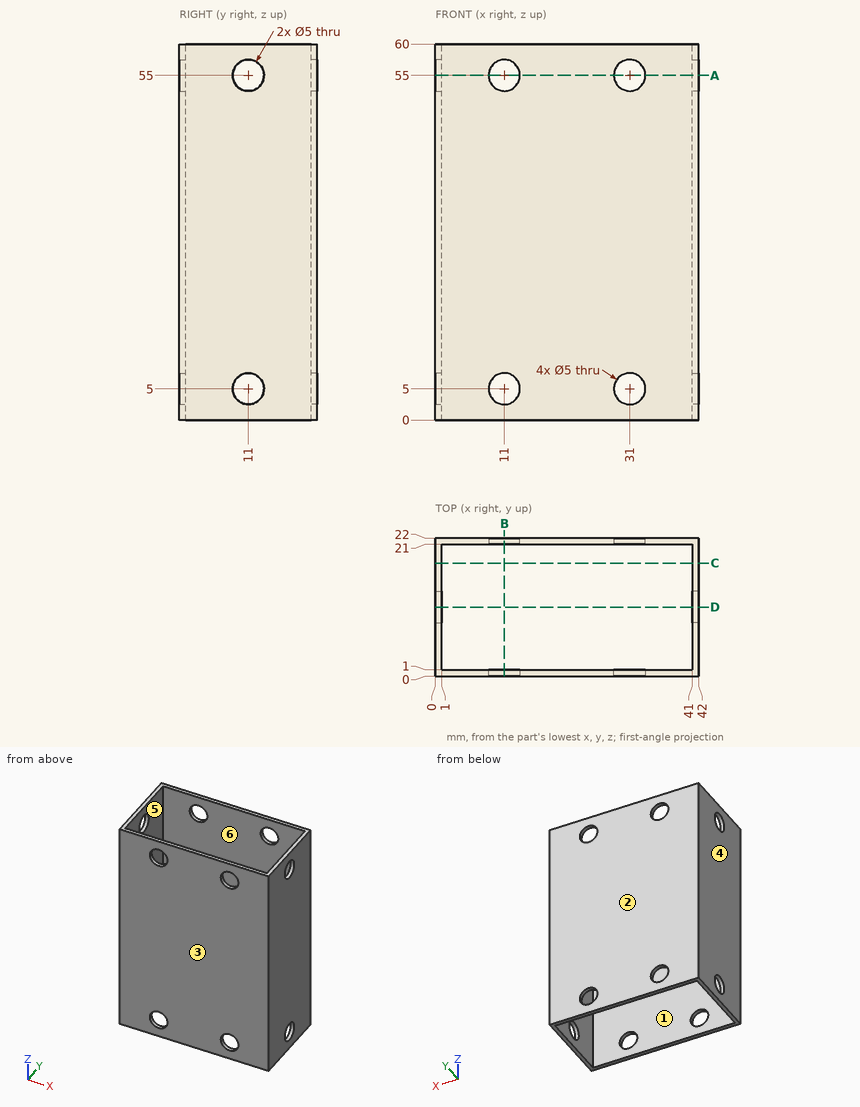
Geometry check sheet. Reference: drawing and pictorial views, mm from the part's lowest x, y, z. A direction names the side the tool comes from. Give positions to 0.01 mm unless a question says otherwise; leave off trailing zeros. Order: outer loops, then holes, each group sorted by start corner. A loop starts at its lowest first (then second) coordinate and runs counter-clockwise, first axis right, second up.
1. Release check for a two-part mould opening along X. For the marked faces 3, 4, 5 and 6 record: pulls with the +X half, pulls with the -X half, needs draft (parallel to the pull), parting line crosses it, or undercut.
2. Access from +Z, -Z, +X, -X, +Y, -Y to the whole of each face (thin tool, end or side, straight path). Record for the marked faces 1 and 2.
3. Thickness scan on L1, parallel to Z at x = 31, y = 21.4; L2, parallel to Y at x = 26, z = 15; L3, parallel to X at y = 15.75, z = 37. Record the ranges inside material, lowest first.
4. Gauge pin test, flat end, axial feed: pin 1 Ø4.5 at (y, z) = (11, 5) entering from +X. Record the tip position at first contact, or that the pin passes through.
5. Section check B-B, the plane x = 11. Enter the section's corners in (y, z).
6. Section check C-C, the plane y = 18. Enter the section's corners in (x, z), and give its area (3 significant figures).
7. Section check D-D, the plane y = 11. Enter the section's corners in (x, z), and give its area (3 significant figures).
8. Section check A-A, the plane z = 55. Give the number of separate pieces and of enclosed holes in the cut face, and give its area (3 significant figures).
Values follow:
1. face 3: needs draft
1. face 4: pulls with the -X half
1. face 5: undercut
1. face 6: undercut
2. face 1: +Z, -Z
2. face 2: +Z, -Z, +X, -X, +Y
3. L1: z = 0 to 2.5, 7.5 to 52.5, 57.5 to 60
3. L2: y = 0 to 1, 21 to 22
3. L3: x = 0 to 1, 41 to 42
4. pin 1: passes through
5. outline: (0, 0) - (1, 0) - (1, 2.5) - (0, 2.5) - close; (0, 7.5) - (1, 7.5) - (1, 52.5) - (0, 52.5) - close; (0, 57.5) - (1, 57.5) - (1, 60) - (0, 60) - close; (21, 0) - (22, 0) - (22, 2.5) - (21, 2.5) - close; (21, 7.5) - (22, 7.5) - (22, 52.5) - (21, 52.5) - close; (21, 57.5) - (22, 57.5) - (22, 60) - (21, 60) - close
6. outline: (0, 0) - (1, 0) - (1, 60) - (0, 60) - close; (41, 0) - (42, 0) - (42, 60) - (41, 60) - close
6. area: 120 mm2
7. outline: (0, 0) - (1, 0) - (1, 2.5) - (0, 2.5) - close; (0, 7.5) - (1, 7.5) - (1, 52.5) - (0, 52.5) - close; (0, 57.5) - (1, 57.5) - (1, 60) - (0, 60) - close; (41, 0) - (42, 0) - (42, 2.5) - (41, 2.5) - close; (41, 7.5) - (42, 7.5) - (42, 52.5) - (41, 52.5) - close; (41, 57.5) - (42, 57.5) - (42, 60) - (41, 60) - close
7. area: 100 mm2
8. separate pieces: 6
8. enclosed holes: 0
8. area: 94.0 mm2
